Input: part model. Units: mm. Frame: model coordinates. Face numbers are marked on the shaded views. A direction names the side the tool comes from. Round coordinates to 2 decimals unless told otherwise and drop trailing zeros. Order: outer loops, then holes, each group sorted by start corner. A loop starts at its lowest first (then second) coordinate and runs counter-clockwise, first axis right, second up. Notation, with made-up numbers: (26.25, -3.75) -> (55.25, -3.75) arc R37 ccw to (55.25, 34.25) -> close; hole circle Ø7 at (-24.5, -12.75). An arc over 180 degrees is marked (long way). Use a Markdown table: item, result.
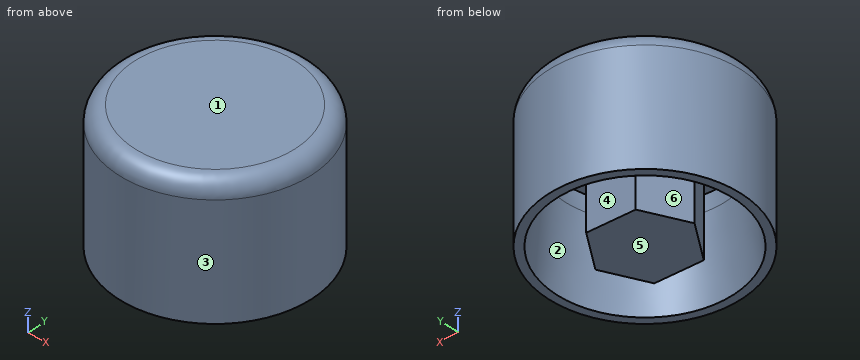
from build123d import *

# Parameters (mm, degrees)
F1_DEPTH = 6
F2_R     = 5
F3_DEPTH = 2
F4_R     = 6
F4_R_2   = 5
F5_DEPTH = 8
F6_R     = 1
F7_SIZE2 = 5
F7_SIZE  = 0.5


with BuildPart() as f1:
    # F0 (on Top) → F1 (new body)
    with BuildSketch(Plane.XY):
        Polygon((1.6334467892, -2.3801648935), (2.8780066576, 0.2245239684), (1.2445598684, 2.6046888619), (-1.6334467892, 2.3801648935), (-2.8780066576, -0.2245239684), (-1.2445598684, -2.6046888619), align=None)
    extrude(amount=F1_DEPTH)

    # F2 (on face) → F3 (join)
    with BuildSketch(Plane.XY.offset(6)):
        Circle(F2_R)
        Polygon((-1.2445598684, -2.6046888619), (-2.8780066576, -0.2245239684), (-1.6334467892, 2.3801648935), (1.2445598684, 2.6046888619), (2.8780066576, 0.2245239684), (1.6334467892, -2.3801648935), align=None, mode=Mode.SUBTRACT)
        Polygon((-1.6334467892, 2.3801648935), (-2.8780066576, -0.2245239684), (-1.2445598684, -2.6046888619), (1.6334467892, -2.3801648935), (2.8780066576, 0.2245239684), (1.2445598684, 2.6046888619), align=None)
    extrude(amount=F3_DEPTH)

    # F4 (on face) → F5 (join)
    with BuildSketch(Plane.XY.offset(8)):
        Circle(F4_R)
        Circle(F4_R_2, mode=Mode.SUBTRACT)
    extrude(amount=-F5_DEPTH)

    # F6
    f6_edges = [f1.edges().sort_by_distance(p)[0] for p in [
        (-6, 0, 8),
    ]]
    fillet(f6_edges, radius=F6_R)

    # F7
    f7_edges = [f1.edges().sort_by_distance(p)[0] for p in [
        (-5, 0, 0),
    ]]
    f7_side = f1.faces().sort_by_distance((-5.830294, 0, 0))[0]
    chamfer(f7_edges, length=F7_SIZE, length2=F7_SIZE2, reference=f7_side)


solid = f1.part
1) Pull-direction query (Y, two-part tool) for the marked faces 1, 2, 3 and 4; classes: +Y half, -Y half, draft (parallel to the pull), parting line (faces both ways), or undercut.
Results found:
| item | result |
|---|---|
| face 1 | draft |
| face 2 | undercut |
| face 3 | parting line |
| face 4 | undercut |
2) Set-up query: the marked faces 5 and 6. Return all of +Z, -Z, +X, -X, +Y, -Y with unobstructed straight access to the full face (end or side cutting, diameter ignored); none if empty.
Results found:
| item | result |
|---|---|
| face 5 | -Z, +X, -X, +Y, -Y |
| face 6 | -Z |
3) Cut plane A-A on z = 2.5. Return loops of the section in (x, y), and give its area (3 significant figures).
Results found:
| item | result |
|---|---|
| outline | circle Ø12 at (0, 0); (-2.88, -0.22) -> (-1.24, -2.6) -> (1.63, -2.38) -> (2.88, 0.22) -> (1.24, 2.6) -> (-1.63, 2.38) -> close; hole circle Ø10.5 at (0, 0) |
| area | 48.2 mm² |
4) Cut plane C-C on y = 0. Return loops of the section in (x, z), and give its area (3 significant figures).
Results found:
| item | result |
|---|---|
| outline | (-6, 0) -> (-5.5, 0) -> (-5, 5) -> (-5, 6) -> (-2.77, 6) -> (-2.77, 0) -> (2.77, 0) -> (2.77, 6) -> (5, 6) -> (5, 5) -> (5.5, 0) -> (6, 0) -> (6, 7) arc R1 ccw to (5, 8) -> (-5, 8) arc R1 ccw to (-6, 7) -> close |
| area | 66.3 mm² |
5) Pin query (flat end, axial travel): pin 1 Ø1.5 at (x, z) = (0.5, 2.5) entering from +Y. Return the tip coordinate at first contact, or that it passes through.
Results found:
| item | result |
|---|---|
| pin 1 | stops at y = 6 |
6) Line query: L1, parallel to Y at x = 2, z = 2; L2, parallel to Y at x = 0, z = 5.65; L3, parallel to X at y = 1, z = 3.5. Output: solid intervals per line, ascending. Write a range as [from, to].
Results found:
| item | result |
|---|---|
| L1 | y = [-5.66, -4.91], [-1.61, 1.5], [4.91, 5.66] |
| L2 | y = [-6, -5], [-2.51, 2.51], [5, 6] |
| L3 | x = [-5.92, -5.05], [-2.29, 2.35], [5.05, 5.92] |
7) Cut plane B-B on x = 0. Return loops of the section in (y, z), and give its area (3 significant figures).
Results found:
| item | result |
|---|---|
| outline | (-6, 0) -> (-5.5, 0) -> (-5, 5) -> (-5, 6) -> (-2.51, 6) -> (-2.51, 0) -> (2.51, 0) -> (2.51, 6) -> (5, 6) -> (5, 5) -> (5.5, 0) -> (6, 0) -> (6, 7) arc R1 ccw to (5, 8) -> (-5, 8) arc R1 ccw to (-6, 7) -> close |
| area | 63.2 mm² |
